Here's how the part is built. I have some questions about the finished solid (model axes, mm). A direction names the side the tool comes from. Coordinates: 2 decimals unless noted, no trailing zeros. Write each loop counter-clockwise with the first axis right and the second up, starting at its lowest first coordinate (ties: lowest second). Pieces come first, ordered by that corner, then holes.
Autodesk Inventor part; units mm, degrees
ref_plane "YZ Plane" through (0, 0, 0) normal (1, 0, 0) x (0, 1, 0)
ref_plane "XZ Plane" through (0, 0, 0) normal (0, 1, 0) x (-1, 0, 0)
ref_plane "XY Plane" through (0, 0, 0) normal (0, 0, 1) x (1, 0, 0)
sketch "Sketch1" plane through (0, 0, 0) normal (0, 1, 0) x (-1, 0, 0)
  line L0 (0, 0) -> (0, 22.8)
  line L1 (0, 22.8) -> (-2, 22.8)
  line L2 (-2, 22.8) -> (-2, 17.8)
  line L3 (-2, 17.8) -> (-3, 17.8)
  line L4 (-3, 17.8) -> (-3, 2.8)
  line L5 (-3, 2.8) -> (-5, 2.8)
  line L6 (-5, 2.8) -> (-5, 0)
  line L7 (-5, 0) -> (0, 0)
  dimension "d0" = 10
  dimension "d1" = 6
  dimension "d2" = 4
  dimension "d3" = 5
  dimension "d4" = 15
  dimension "d5" = 2.8
revolve "Revolution1" add sketch "Sketch1" angle 360 about axis through (0, 0, 0) along (0, 0, 1)
thread "Thread1"
sketch "Sketch2" plane through (0, 0, 0) normal (0, 0, -1) x (-1, 0, 0)
  line L0 (0, 1.4434) -> (1.25, 0.7217)
  line L1 (1.25, 0.7217) -> (1.25, -0.7217)
  line L2 (1.25, -0.7217) -> (0, -1.4434)
  line L3 (0, -1.4434) -> (-1.25, -0.7217)
  line L4 (-1.25, -0.7217) -> (-1.25, 0.7217)
  line L5 (-1.25, 0.7217) -> (0, 1.4434)
  point P0 (0, 0)
  point P1 (0, 0)
  dimension "d9" = 2.5
extrude "Extrusion1" cut sketch "Sketch2" against normal blind 2
chamfer "Chamfer1" distance 0.43 angle 45 1 edges at (-2, 0, 22.8)
properties part number "DBTSY4-15-5-DHC" material "Stainless Steel AISI 304"
1. I want a section at D-D (z = 20.25). List the corners of the cut face in (x, y) for me.
2. I want a section at C-C (x = 4). List the corners of the cut face in (y, z) for me.
3. If I drill on line 1 (Z direction, x = 3, y = 1.5); line 2 (Z direction, x = -0.25, y = 0); line 3 (X direction, y = 2, z = 13.25), over which ranges is the centre line in solid material (lowest first)?
4. Thinking about a two-plate mould opening in X: for faces 1 (the face through (0.63, 1.08, 0.99)), 2 (the face through (-1.08, 4.88, 1.38)), 3 (the face through (0, 0, 22.8)), 4 (the face through (-0.63, -1.08, 0.99)), which applies, pulls with the +X half, pulls with the -X half, needs draft (parallel to the pull), parting line crosses it, or undercut?
5. For pin 1 Ø3 at (y, z) = (3.5, 13.5) entering from -X; pin 2 Ø0.8 at (x, y) = (0.5, 0.5) entering from -Z; pin 3 Ø1.5 at (x, y) = (-3.5, 2) entering from +Z, each with a flat end and sliding along its axis, tell me the tip position at first contact or that it passes through.
6. On a 3-axis mill with a long thin cutter (end or side, diameter ignored), from which of +Z, -Z, +X, -X, +Y, -Y can I reach the whole of each face in a straight line? I mean faces 5 (the face through (-1.25, 0, 1)), 6 (the face through (1, -2, 17.8)), 7 (the face through (1.04, -1.04, 0)). Say none if no direction works.
7. I want a section at A-A (y = 0). List the corners of the cut face in (x, z) for me.
8. I want a section at B-B (z = 11.75). List the corners of the cut face in (x, y) for me.
Response values:
1. outline: circle Ø4 at (0, 0)
2. outline: (-3, 0) - (3, 0) - (3, 2.8) - (-3, 2.8) - close
3. line 1: z = 0 to 2.8
3. line 2: z = 2 to 22.8
3. line 3: x = -2.24 to 2.24
4. face 1: undercut
4. face 2: parting line crosses it
4. face 3: needs draft
4. face 4: undercut
5. pin 1: stops at x = -2.24
5. pin 2: stops at z = 2
5. pin 3: stops at z = 2.8
6. face 5: -Z
6. face 6: +Z
6. face 7: -Z, +X, -X, +Y, -Y
7. outline: (-5, 0) - (-1.25, 0) - (-1.25, 2) - (1.25, 2) - (1.25, 0) - (5, 0) - (5, 2.8) - (3, 2.8) - (3, 17.8) - (2, 17.8) - (2, 22.37) - (1.57, 22.8) - (-1.57, 22.8) - (-2, 22.37) - (-2, 17.8) - (-3, 17.8) - (-3, 2.8) - (-5, 2.8) - close
8. outline: circle Ø6 at (0, 0)
